```python
from build123d import *


with BuildPart() as part:
    # Esquisse1 → Base-Révolution (revolve)
    with BuildSketch(Plane.XY, mode=Mode.PRIVATE) as base_r_volution_sk:
        Polygon((0, 15), (32, 15), (38, 16), (299, 16), (304, 17), (304, 17.5), (305.5, 17.5), (305.5, 15.770294146), (299.14852927, 14.5), (38.124143795, 14.5), (32.124143795, 13.5), (0, 13.5), align=None)
    revolve(base_r_volution_sk.sketch.rotate(Axis((0, 0, 0), (1, 0, 0)), 90), axis=Axis((0, 0, 0), (1, 0, 0)))


solid = part.part
```
Read the model definition and answer for the solid it produces. Units are mm, in the model's axes. A direction names the side the tool comes from. Give positions to 0.01 mm unless a question says otherwise; leave off trailing zeros. Loops run counter-clockwise (first coordinate to the right, second up) from the corner with the lowest first, then second, coordinate; pieces in that order, holes last.
Item 1: The part is cut by section C-C (x = 26.5). Write down the section's boundary in (y, z).
Item 2: Find the intervals of material crossed by line 1 along Y through (x, z) = (14, 0); line 2 along Y through (x, z) = (234, -0.5); line 3 along Z through (x, y) = (286, -12.5), in increasing order.
Item 3: The part is cut by section D-D (x = 164.5). Write down the section's boundary in (y, z).
Item 4: Each of these flat-tipped pins is pushed along its axis until it touches: pin 1 Ø12 at (y, z) = (-13.5, -1.5) entering from -X; pin 2 Ø10 at (x, y) = (131, -3) entering from +Z; pin 3 Ø5 at (x, z) = (173, 5.5) entering from +Y; pin 4 Ø8 at (x, z) = (87.5, 1) entering from -Y. Where does it stop, or does it pass through?
Item 5: The part is cut by section A-A (y = 0). Write down the section's boundary in (x, z), and give its area (3 significant figures).
Item 6: The mould has two halves that part along Y. Classify faces 1 (the conical face through (299.31, 15.68, -3.48)), 2 (the flat face through (304, -17, 3)), 3 (the cylindrical face through (166.809, 12.864, 6.691)): released by +Y, released by -Y, zero draft, split by the parting line, or undercut.
Item 7: For faces 4 (the cylindrical face through (304.76, 17.084, -3.794)), 5 (the cylindrical face through (16.22, -12.65, 8.06)), determine the directions among +Z, -Z, +X, -X, +Y, -Y from which every point of the face is accessible in a straight line to the end or side of a thin tool.
Taken from the geometry:
1. outline: circle Ø30 at (0, 0); hole circle Ø27 at (0, 0)
2. line 1: y = -15 to -13.5, 13.5 to 15
2. line 2: y = -15.99 to -14.49, 14.49 to 15.99
2. line 3: z = -9.99 to -7.35, 7.35 to 9.99
3. outline: circle Ø32 at (0, 0); hole circle Ø29 at (0, 0)
4. pin 1: stops at x = 0
4. pin 2: stops at z = 16
4. pin 3: stops at y = 15.72
4. pin 4: stops at y = -16
5. outline: (0, -15) - (32, -15) - (38, -16) - (299, -16) - (304, -17) - (304, -17.5) - (305.5, -17.5) - (305.5, -15.77) - (299.15, -14.5) - (38.12, -14.5) - (32.12, -13.5) - (0, -13.5) - close; (0, 13.5) - (32.12, 13.5) - (38.12, 14.5) - (299.15, 14.5) - (305.5, 15.77) - (305.5, 17.5) - (304, 17.5) - (304, 17) - (299, 16) - (38, 16) - (32, 15) - (0, 15) - close
5. area: 918 mm2
6. face 1: split by the parting line
6. face 2: zero draft
6. face 3: undercut
7. face 4: +X, -X
7. face 5: -X
